Work out the finished part from the listing and answer in its coordinate system (mm). A direction names the side the tool comes from. Coordinates: 2 decimals unless noted, no trailing zeros. Order: outer loops, then holes, each group sorted by start corner. A loop starts at its lowest first (then second) coordinate and runs counter-clockwise, first axis right, second up. Notation, with made-up numbers: M -22.75,26 L 5.25,26 A20 ccw 5.25,42 Z; hole C 85.5,-24 d7. An arc over 180 degrees is marked long. Use a Markdown table: item, result.
from build123d import *

# Parameters (mm, degrees)
SKETCH_R     = 1.778
PAD_DEPTH    = 21.59
POCKET_DEPTH = 12.7


with BuildPart() as part:
    # Sketch → Pad (new body)
    with BuildSketch(Plane.XY):
        with BuildLine():
            ThreePointArc((16.3195, -28.266203), (32.639, 0), (16.3195, 28.266203))
            Line((16.3195, 28.266203), (17.4625, 30.245937))
            ThreePointArc((30.56252, 16.902308), (24.922154, 24.467159), (17.4625, 30.245937))
            ThreePointArc((34.218529, 6.989129), (39.797707, 14.677509), (30.56252, 16.902308))
            ThreePointArc((34.218529, -6.989129), (34.925, 0), (34.218529, 6.989129))
            ThreePointArc((30.56252, -16.902308), (39.797707, -14.677509), (34.218529, -6.989129))
            ThreePointArc((17.4625, -30.245937), (24.922154, -24.467159), (30.56252, -16.902308))
            Line((16.3195, -28.266203), (17.4625, -30.245937))
        make_face()
        with Locations((34.43574, 12.7)):
            Circle(SKETCH_R, mode=Mode.SUBTRACT)
        with Locations((34.43574, -12.7)):
            Circle(SKETCH_R, mode=Mode.SUBTRACT)
    extrude(amount=PAD_DEPTH)

    # Sketch001 → Pocket (cut)
    with BuildSketch(Plane.XY):
        with BuildLine():
            ThreePointArc((34.218529, 6.989129), (39.797707, 14.677509), (30.56252, 16.902308))
            ThreePointArc((34.218529, 6.989129), (32.767573, 12.084775), (30.56252, 16.902308))
        make_face()
        with BuildLine():
            ThreePointArc((30.56252, -16.902308), (39.797707, -14.677509), (34.218529, -6.989129))
            ThreePointArc((30.56252, -16.902308), (32.767573, -12.084775), (34.218529, -6.989129))
        make_face()
    extrude(amount=POCKET_DEPTH, mode=Mode.SUBTRACT)


solid = part.part
(1) Determine the mould class of faces 4 (the flat face through (33, 2, 0)), 5 (the cylindrical face through (32.635, -0.478, 10.644)), 6 (the cylindrical face through (39.85, 14.53, 17.08)) for opening direction X: pulls with the +X half, pulls with the -X half, needs draft (parallel to the pull), parting line crosses it, or undercut.
Conclusion:
| item | result |
|---|---|
| face 4 | needs draft |
| face 5 | pulls with the -X half |
| face 6 | undercut |
(2) A cutting plane is placed at A-A (x = 21.5). Determine the outline of the cut face in (y, z), then the cut area to 3 significant figures.
Conclusion:
| item | result |
|---|---|
| outline | M -27.52,0 L -24.56,0 L -24.56,21.59 L -27.52,21.59 Z; M 24.56,0 L 27.52,0 L 27.52,21.59 L 24.56,21.59 Z |
| area | 128 mm2 |
(3) Which of the six approach directions +Z, -Z, +X, -X, +Y, -Y give full straight-line access (tool end or side, diameter ignored) to faces 1 (the flat face through (36.4, -12.6, 12.7)), 2 (the flat face through (36.4, 12.8, 12.7)), 3 (the flat face through (16.88, 29.24, 10.64))?
Conclusion:
| item | result |
|---|---|
| face 1 | -Z, +X, -Y |
| face 2 | -Z, +X, +Y |
| face 3 | +Z, -Z, -X, +Y |
(4) A cutting plane is placed at B-B (y = -12.7). Determine the outline of the cut face in (x, z).
Conclusion:
| item | result |
|---|---|
| outline | M 30.07,0 L 32.53,0 L 32.53,12.7 L 32.66,12.7 L 32.66,21.59 L 30.07,21.59 Z; M 36.21,12.7 L 40.15,12.7 L 40.15,21.59 L 36.21,21.59 Z |
(5) Given P1, Ø1.5, axis at y = 24, z = 18.5, coming from the -X side; P2, Ø3, axis at y = 17, z = 12, coming from the -X side; P3, Ø8, axis at y = -11.5, z = 8.5, coming from the -X side; P4, Ø2, axis at x = 34.44, y = 12.7, coming from the +Z side, each flat-ended and moving along its own axis, determine where each tip first touches the part or whether it passes through.
Conclusion:
| item | result |
|---|---|
| P1 | x = 21.28 |
| P2 | x = 26.89 |
| P3 | x = 28.72 |
| P4 | through |
(6) A cutting plane is placed at D-D (x = 31.25). Determine the outline of the cut face in (y, z), then the cut area to 3 significant figures.
Conclusion:
| item | result |
|---|---|
| outline | M -17.44,12.7 L -15.59,12.7 L -15.59,0 L -9.42,0 L -9.42,21.59 L -17.44,21.59 Z; M 9.42,0 L 15.59,0 L 15.59,12.7 L 17.44,12.7 L 17.44,21.59 L 9.42,21.59 Z |
| area | 300 mm2 |
(7) Straight lines are drawn through the part: L1, parallel to Y at x = 33, z = 16.5; L2, parallel to Y at x = 33.5, z = 20.25; L3, parallel to Z at x = 33.75, y = 16.5. For each, find the intervals that lie inside material, in ascending order.
Conclusion:
| item | result |
|---|---|
| L1 | -18.23 to -13.75, -11.65 to 11.65, 13.75 to 18.23 |
| L2 | -18.34 to -14.21, -11.19 to 11.19, 14.21 to 18.34 |
| L3 | 12.7 to 21.59 |
